Can you work these out from the model? Positions are in its coordinate system, mm. A direction names the side the tool comes from. Round coordinates to 2 decimals unless told otherwise and drop trailing zeros. Loops run counter-clockwise (first coordinate to the right, second up) from the corner with the lowest first, then second, coordinate; pieces in that order, holes last.
from build123d import *

# Parameters (mm, degrees)
SKETCH1_W                 = 9.8
SKETCH1_H                 = 3.5
BASE_DEPTH                = 7
SKETCH2_W                 = 9.8
SKETCH2_H                 = 13.6
PCB_CUTOUT_DEPTH          = 3
SKETCH5_R                 = 1.4
SCREW_HOLES_DEPTH         = 28.14498112
SKETCH6_W                 = 9.8
SKETCH6_H                 = 4
PIN_HEADERS_OPENING_DEPTH = 3.5
F_1MM_EDGE_FILLETS_R      = 1


with BuildPart() as part:
    # Sketch1 → Base (new body)
    with BuildSketch(Plane(origin=(0, 0, 0), x_dir=(1, 0, 0), z_dir=(0, 1, 0))):
        Polygon((-8.9, 10.8), (-8.9, 5), (-23.9, 5), (-23.9, -5), (-8.9, -5), (-8.9, -10.8), (8.9, -10.8), (8.9, -5), (23.9, -5), (23.9, 5), (8.9, 5), (8.9, 10.8), (0, 10.8), align=None)
        with Locations((0, -5.05)):
            Rectangle(SKETCH1_W, SKETCH1_H, mode=Mode.SUBTRACT)
    extrude(amount=BASE_DEPTH)

    # Sketch2 → PCB Cutout (cut)
    with BuildSketch(Plane(origin=(0, 7, 0), x_dir=(1, 0, 0), z_dir=(0, 1, 0))):
        Rectangle(SKETCH2_W, SKETCH2_H)
    extrude(amount=-PCB_CUTOUT_DEPTH, mode=Mode.SUBTRACT)

    # Sketch5 → Screw Holes (cut, through all)
    with BuildSketch(Plane.XZ):
        with Locations(Location((-20.4, 0, 0), (0, 0, 270))):
            Circle(SKETCH5_R)
        with Locations(Location((20.4, 0, 0), (0, 0, 90))):
            Circle(SKETCH5_R)
    extrude(amount=-SCREW_HOLES_DEPTH, mode=Mode.SUBTRACT)

    # Sketch6 → Pin Headers Opening (cut)
    with BuildSketch(Plane.XZ):
        with Locations((0, 8.8)):
            Rectangle(SKETCH6_W, SKETCH6_H)
    extrude(amount=-PIN_HEADERS_OPENING_DEPTH, mode=Mode.SUBTRACT)

    # 1mm Edge Fillets
    f_1mm_edge_fillets_edges = [part.edges().sort_by_distance(p)[0] for p in [
        (0, 0, -10.8),
        (8.9, 0, -7.9),
        (16.4, 0, -5),
        (23.9, 0, 0),
        (16.4, 0, 5),
        (8.9, 0, 7.9),
        (-6.9, 0, 10.8),
        (-8.9, 0, 7.9),
        (-16.4, 0, 5),
        (-23.9, 0, 0),
        (-16.4, 0, -5),
        (-8.9, 0, -7.9),
        (8.9, 3.5, -10.8),
        (8.9, 3.5, -5),
        (23.9, 3.5, -5),
        (23.9, 3.5, 5),
        (8.9, 3.5, 5),
        (8.9, 3.5, 10.8),
        (-8.9, 3.5, 10.8),
        (-8.9, 3.5, 5),
        (-23.9, 3.5, 5),
        (-23.9, 3.5, -5),
        (-8.9, 3.5, -5),
        (-8.9, 3.5, -10.8),
        (6.9, 0, 10.8),
    ]]
    fillet(f_1mm_edge_fillets_edges, radius=F_1MM_EDGE_FILLETS_R)


solid = part.part
(1) If we mould it in two halves opening along X, with no side actions, what happens to faces 6 (the flat face through (4.9, 4.2, 1.9)), 7 (the flat face through (-6, 7, 0)), 8 (the cylindrical face through (-9.185, 4.042, 5.301))? For each: released by +X, released by -X, zero draft, split by the parting line, or undercut.
Worked answers:
face 6: undercut
face 7: zero draft
face 8: released by -X
(2) If we section it at C-C, the plane z = 0: List the corners of the cut face in (x, y) for me, then the cut area to 3 significant figures.
Worked answers:
outline: (-23.9, 1) arc R1 ccw to (-22.9, 0) - (-21.8, 0) - (-21.8, 7) - (-23.9, 7) - close; (-19, 0) - (19, 0) - (19, 7) - (4.9, 7) - (4.9, 4) - (-4.9, 4) - (-4.9, 7) - (-19, 7) - close; (21.8, 0) - (22.9, 0) arc R1 ccw to (23.9, 1) - (23.9, 7) - (21.8, 7) - close
area: 266 mm2
(3) If I drill on line 1 (X direction, y = 3.5, z = 0); line 2 (X direction, y = 5.25, z = 0); line 3 (Z direction, x = 20.4, y = 5.25), over which ranges is the centre line in solid material (lowest first)?
Worked answers:
line 1: x = -23.9 to -21.8, -19 to 19, 21.8 to 23.9
line 2: x = -23.9 to -21.8, -19 to -4.9, 4.9 to 19, 21.8 to 23.9
line 3: z = -5 to -1.4, 1.4 to 5
(4) If we section it at B-B, the plane x = 20.4: List the corners of the cut face in (y, z) for me.
Worked answers:
outline: (0, -4) arc R1 ccw to (1, -5) - (7, -5) - (7, -1.4) - (0, -1.4) - close; (0, 1.4) - (7, 1.4) - (7, 5) - (1, 5) arc R1 ccw to (0, 4) - close
(5) If we section it at D-D, the plane z = 9: List the corners of the cut face in (x, y) for me.
Worked answers:
outline: (-8.9, 1) arc R1 ccw to (-7.9, 0) - (-4.9, 0) - (-4.9, 3.5) - (4.9, 3.5) - (4.9, 0) - (7.9, 0) arc R1 ccw to (8.9, 1) - (8.9, 7) - (-8.9, 7) - close
(6) If we section it at A-A, the plane y = 1.75: State how many separate pieces and enclosed holes the cut face has, then the cut area to 3 significant figures.
Worked answers:
separate pieces: 1
enclosed holes: 2
area: 598 mm2
(7) Will these pins go through, and if not, where does the flat tip stop? P1, Ø3, axis at x = -1.5, y = 1.5, coming from the +Z side; P2, Ø3, axis at x = 18, y = 4.5, coming from the +Z side; P3, Ø3, axis at x = 13.5, y = 3, coming from the -Z side; P4, Ø1.7, axis at x = 20.4, z = 0, coming from the -Y side.
Worked answers:
P1: stops at z = 3.3
P2: stops at z = 5
P3: stops at z = -5
P4: passes through
(8) For faces 1 (the cylindrical face through (16.491, 0.301, 4.715)), 2 (the cylindrical face through (-16.309, 0.301, 4.715)), 3 (the flat face through (0, 5, 6.8)), 4 (the cylindrical face through (8.615, 0.301, -7.927)), 5 (the flat face through (-16, 4, 5)), which set-ups out of +Z, -Z, +X, -X, +Y, -Y let a thin tool reach every point of the face, with its end or its side?
Worked answers:
face 1: +Z, +X, -Y
face 2: +Z, -X, -Y
face 3: +Y, -Y
face 4: -Z, +X, -Y
face 5: +Z, -X, +Y, -Y
